Part model, mm, in its own coordinate system. A direction names the side the tool comes from. Give positions to 0.01 mm unless a question says otherwise; leave off trailing zeros. Write each loop counter-clockwise with the first axis right and the second up, starting at its lowest first coordinate (ties: lowest second). Pieces come first, ordered by that corner, then holes. Notation, with made-up numbers: M 80.25,74.5 L 105.25,74.5 A18 cw 105.25,102.5 Z; hole C -24.5,-29 d8. An arc over 180 degrees is marked long. Answer as CSV lines item,"result". Start each with the question number.
1) Slice it at C-C, the plane x = 9.25. Give the cut face in (y, z) (3 decimals).
2) Pin check, flat tips, straight feed: pin 1 Ø5 at (y, z) = (185.772, 14.287) entering from -X; pin 2 Ø8.5 at (x, y) = (14.287, 160.312) entering from +Z (3 decimals); pin 3 Ø1.5 at (y, z) = (114.5, 11) entering from +X (3 decimals). Stop position of each tip, or through.
3) Wall check: line 1 along Z through (x, y) = (24.25, 144) (3 decimals). Give the ranges that are in metal, low to high. Write a range as from..to.
4) Tool access for faces 1 (the cylindrical face through (1.57, 183.03, 12.54)), 2 (the flat face through (14, 99, 3.175)): list every direction of +Z, -Z, +X, -X, +Y, -Y with a clear straight run to the whole face (end or side of a thin tool).
5) Slice it at A-A, the plane z = 13. Give the cut face in (x, y) (3 decimals), plus the area to 3 significant figures.
6) Mould opens along Y. For faces 3 (the flat face through (3.175, 99, 14)), 4 (the cylindrical face through (1.565, 13.091, 16.866)), 5 (the flat face through (2, 200, 7)) say: pulls with the +Y half, pulls with the -Y half, needs draft (parallel to the pull), parting line crosses it, or undercut.
7) Slice it at B-B, the plane y = 178. Give the cut face in (x, z) (3 decimals).
Autodesk Fusion 360 part; units mm, degrees
sketch "Sketch1" plane through (0, 0, 0) normal (0, 1, 0) x (1, 0, 0)
  line L0 (0, -25.4) -> (0, 0)
  line L1 (0, 0) -> (25.4, 0)
  line L2 (12.7, -12.7) -> (11.05, -11.05) construction
  line L3 (3.175, -25.4) -> (3.175, -3.175)
  line L4 (3.175, -3.175) -> (25.4, -3.175)
  line L5 (25.4, -3.175) -> (25.4, 0)
  line L6 (0, -25.4) -> (3.175, -25.4)
  dimension "d1" = 25.4
  dimension "d2" = 25.4
  dimension "d13" = 3.175
extrude "Extrude1" add sketch "Sketch1" along normal blind 200
hole "Hole3" at (3.175, 11.113, 14.287) direction (-1, 0, 0) diameter 6.5 end through all
hole "Hole4" at (3.175, 185.772, 14.287) direction (-1, 0, 0) diameter 6.5 depth 30 tip angle 118
hole "Hole5" at (14.287, 160.312, 3.175) direction (0, 0, -1) diameter 6.5 depth 30 tip angle 118
Found:
1,outline,"M 0,0 L 200,0 L 200,3.175 L 0,3.175 Z"
2,pin 1,"through"
2,pin 2,"z = 3.175"
2,pin 3,"x = 3.175"
3,line 1,"0..3.175"
4,face 1,"+X, -X"
4,face 2,"+Z, +X, +Y, -Y"
5,outline,"M 0,0 L 3.175,0 L 3.175,8.129 L 0,8.129 Z; M 0,14.097 L 3.175,14.097 L 3.175,182.788 L 0,182.788 Z; M 0,188.756 L 3.175,188.756 L 3.175,200 L 0,200 Z"
5,area,"597 mm²"
6,face 3,"needs draft"
6,face 4,"undercut"
6,face 5,"pulls with the +Y half"
7,outline,"M 0,0 L 25.4,0 L 25.4,3.175 L 3.175,3.175 L 3.175,25.4 L 0,25.4 Z"
